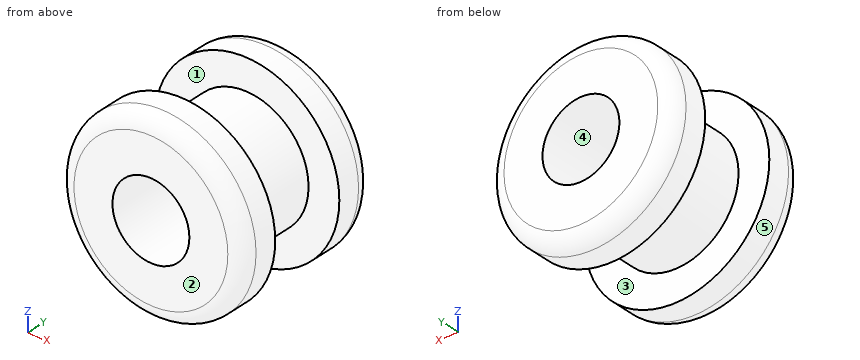
Autodesk Inventor part; units mm, degrees
ref_plane "YZ Plane" through (0, 0, 0) normal (1, 0, 0) x (0, 1, 0)
ref_plane "XZ Plane" through (0, 0, 0) normal (0, 1, 0) x (-1, 0, 0)
ref_plane "XY Plane" through (0, 0, 0) normal (0, 0, 1) x (1, 0, 0)
sketch "Эскиз1" plane through (0, 0, 0) normal (0, 1, 0) x (-1, 0, 0)
  circle A0 centre (0, 0) radius 2
  dimension "d0" = 4
extrude "Выдавливание1" add sketch "Эскиз1" along normal blind 5
sketch "Эскиз2" plane through (0, 5, 0) normal (0, 1, 0) x (1, 0, 0)
  circle A0 centre (0, 0) radius 3
  dimension "d3" = 6
extrude "Выдавливание2" add sketch "Эскиз2" against normal blind 1.25
sketch "Эскиз3" plane through (0, 0, 0) normal (0, -1, 0) x (1, 0, 0)
  circle A0 centre (0, 0) radius 3
extrude "Выдавливание3" add sketch "Эскиз3" against normal blind 1.25
sketch "Эскиз4" plane through (0, 0, 0) normal (0, -1, 0) x (1, 0, 0)
  circle A0 centre (0, 0) radius 1.25
  dimension "d12" = 2.5
extrude "Выдавливание4" cut sketch "Эскиз4" against normal blind 12
fillet "Сопряжение1" radius 0.5 2 edges at (-3, 0, 0) (-3, 5, 0)
properties part number "vtulka_servo"
CAD build for the part. Positions are in the model's coordinates, mm. Face numbers are marked on the shaded views. A direction names the side the tool comes from. Give positions to 0.01 mm unless a question says otherwise; leave off trailing zeros. Order: outer loops, then holes, each group sorted by start corner. A loop starts at its lowest first (then second) coordinate and runs counter-clockwise, first axis right, second up.
(1) Saw through at A-A, the plane x = 0. Give the cut face in (y, z).
(2) Tool access for the marked faces 1 and 2: list every direction of +Z, -Z, +X, -X, +Y, -Y with a clear straight run to the whole face (end or side of a thin tool).
(3) Drill centre lines: L1, parallel to Z at x = 0, y = 1; L2, parallel to Z at x = 0, y = 3.45; L3, parallel to Y at x = 0, z = 2.45. Where is each one in solid material? Low to high.
(4) Saw through at B-B, the plane z = 0. Give the cut face in (x, y).
(5) Mould opens along X. For the marked faces 3, 4 and 5 say: released by +X, released by -X, zero draft, split by the parting line, or undercut.
(6) Saw through at D-D, the plane y = 3.5. Give the cut face in (x, z).
(7) Saw through at C-C, the plane y = 4.1. Give the cut face in (x, z), then the cut area to 3 significant figures.
(8) Flat gauge pin, fed straight in: pin 1 (1.5 mm diameter, centred on y = 3.5, z = -2, fed in from +X). Where does the tip first touch, or does it go through?
Results found:
1. outline: (0, -2.5) arc R0.5 ccw to (0.5, -3) - (1.25, -3) - (1.25, -2) - (3.75, -2) - (3.75, -3) - (4.5, -3) arc R0.5 ccw to (5, -2.5) - (5, -1.25) - (0, -1.25) - close; (0, 1.25) - (5, 1.25) - (5, 2.5) arc R0.5 ccw to (4.5, 3) - (3.75, 3) - (3.75, 2) - (1.25, 2) - (1.25, 3) - (0.5, 3) arc R0.5 ccw to (0, 2.5) - close
2. face 1: none
2. face 2: +Z, -Z, +X, -X, -Y
3. L1: z = -3 to -1.25, 1.25 to 3
3. L2: z = -2 to -1.25, 1.25 to 2
3. L3: y = 0 to 1.25, 3.75 to 5
4. outline: (-3, 0.5) arc R0.5 ccw to (-2.5, 0) - (-1.25, 0) - (-1.25, 5) - (-2.5, 5) arc R0.5 ccw to (-3, 4.5) - (-3, 3.75) - (-2, 3.75) - (-2, 1.25) - (-3, 1.25) - close; (1.25, 0) - (2.5, 0) arc R0.5 ccw to (3, 0.5) - (3, 1.25) - (2, 1.25) - (2, 3.75) - (3, 3.75) - (3, 4.5) arc R0.5 ccw to (2.5, 5) - (1.25, 5) - close
5. face 3: zero draft
5. face 4: undercut
5. face 5: split by the parting line
6. outline: circle Ø4 at (0, 0); hole circle Ø2.5 at (0, 0)
7. outline: circle Ø6 at (0, 0); hole circle Ø2.5 at (0, 0)
7. area: 23.4 mm2
8. pin 1: stops at x = 2.71
